Part model, mm, in its own coordinate system. A direction names the side the tool comes from. Round coordinates to 2 decimals unless told otherwise and drop trailing zeros. Loops run counter-clockwise (first coordinate to the right, second up) from the corner with the lowest first, then second, coordinate; pieces in that order, holes last.
1) Band-saw the part on C-C, the plane z = 3.5. Write the cut outline in (x, y).
2) Probe line 1 (X direction, y = -19.05, z = 6.25); line 2 (Y direction, x = 0, z = 9); line 3 (Z direction, x = 21.5, y = 34). List the from-to ranges inside material, lowest first.
3) Drop flat-ended pins along their axis: P1, Ø8, axis at x = -27.5, y = -29.5, coming from the -Z side; P2, Ø11.5, axis at x = 15, z = -11.5, coming from the -Y side. Give the stop position or say it passes through.
4) Mould opens along Y. For faces 4 (the flat face through (0, -50.8, 6)), 5 (the flat face through (38.1, 21, 1)), 6 (the cylindrical face through (-4.13, -37.647, 6.261)), 7 (the flat face through (-1, 50.8, -12)) say: +Y half, -Y half, draft (parallel to the pull), parting line (faces both ways), or undercut.
5) 3-axis set-ups, long thin cutter, end or side, ignore diameter. For faces 1 (the flat face through (-1, 25.4, -19)), 2 (the cylindrical face through (-30.86, -43.16, 6.44)), 3 (the flat face through (28, 38, -19.05)): which of +Z, -Z, +X, -X, +Y, -Y reach the whole face in a straight line?
6) Band-saw the part on A-A, the plane x = 0. Write the cut outline in (y, z), then the cut area to 3 significant figures.
7) Band-saw the part on B-B, the plane y = -19.05. Write the cut outline in (x, z), then the cut area to 3 significant figures.
8) Band-saw the part on D-D, the plane y = 41. Write the cut outline in (x, z), then the cut area to 3 significant figures.
from build123d import *

# Parameters (mm, degrees)
F0_W     = 76.2
F0_H     = 101.6
F1_DEPTH = 12.7
F2_R     = 19.05
F3_DEPTH = 25.4
F4_W     = 76.2
F4_H     = 25.4
F5_DEPTH = 38.1
F6_W     = 19.05
F6_H     = 19.05
F7_DEPTH = 25.4
F8_R     = 25.4


with BuildPart() as f1:
    # F0 (on Top) → F1 (new body)
    with BuildSketch(Plane.XY):
        Rectangle(F0_W, F0_H)
    extrude(amount=F1_DEPTH)

    # F2 (on Top) → F3 (cut)
    with BuildSketch(Plane.XY):
        with Locations((0, -19.05)):
            Circle(F2_R)
    extrude(amount=F3_DEPTH, mode=Mode.SUBTRACT)

    # F4 (on Top) → F5 (join)
    with BuildSketch(Plane.XY):
        with Locations((0, 38.1)):
            Rectangle(F4_W, F4_H)
    extrude(amount=-F5_DEPTH)

    # F6 (on face) → F7 (cut)
    with BuildSketch(Plane.XZ.offset(-25.4)):
        with Locations((28.575, -28.575)):
            Rectangle(F6_W, F6_H)
    extrude(amount=-F7_DEPTH, mode=Mode.SUBTRACT)

    # F8
    f8_edges = [f1.edges().sort_by_distance(p)[0] for p in [
        (38.1, -50.8, 6.35),
        (-38.1, -50.8, 6.35),
    ]]
    fillet(f8_edges, radius=F8_R)


solid = f1.part
Reported:
1. outline: (-38.1, -25.4) arc R25.4 ccw to (-12.7, -50.8) - (12.7, -50.8) arc R25.4 ccw to (38.1, -25.4) - (38.1, 50.8) - (-38.1, 50.8) - close; hole circle Ø38.1 at (0, -19.05)
2. line 1: x = -38.1 to -19.05, 19.05 to 38.1
2. line 2: y = -50.8 to -38.1, 0 to 50.8
2. line 3: z = -19.05 to 12.7
3. P1: stops at z = 0
3. P2: stops at y = 25.4
4. face 4: -Y half
4. face 5: draft
4. face 6: undercut
4. face 7: +Y half
5. face 1: -Z, +X, -X, -Y
5. face 2: +Z, -Z, -X, -Y
5. face 3: -Z, +X, +Y, -Y
6. outline: (-50.8, 0) - (-38.1, 0) - (-38.1, 12.7) - (-50.8, 12.7) - close; (0, 0) - (25.4, 0) - (25.4, -38.1) - (50.8, -38.1) - (50.8, 12.7) - (0, 12.7) - close
6. area: 1,770 mm2
7. outline: (-38.1, 0) - (-19.05, 0) - (-19.05, 12.7) - (-38.1, 12.7) - close; (19.05, 0) - (38.1, 0) - (38.1, 12.7) - (19.05, 12.7) - close
7. area: 484 mm2
8. outline: (-38.1, -38.1) - (19.05, -38.1) - (19.05, -19.05) - (38.1, -19.05) - (38.1, 12.7) - (-38.1, 12.7) - close
8. area: 3,510 mm2
